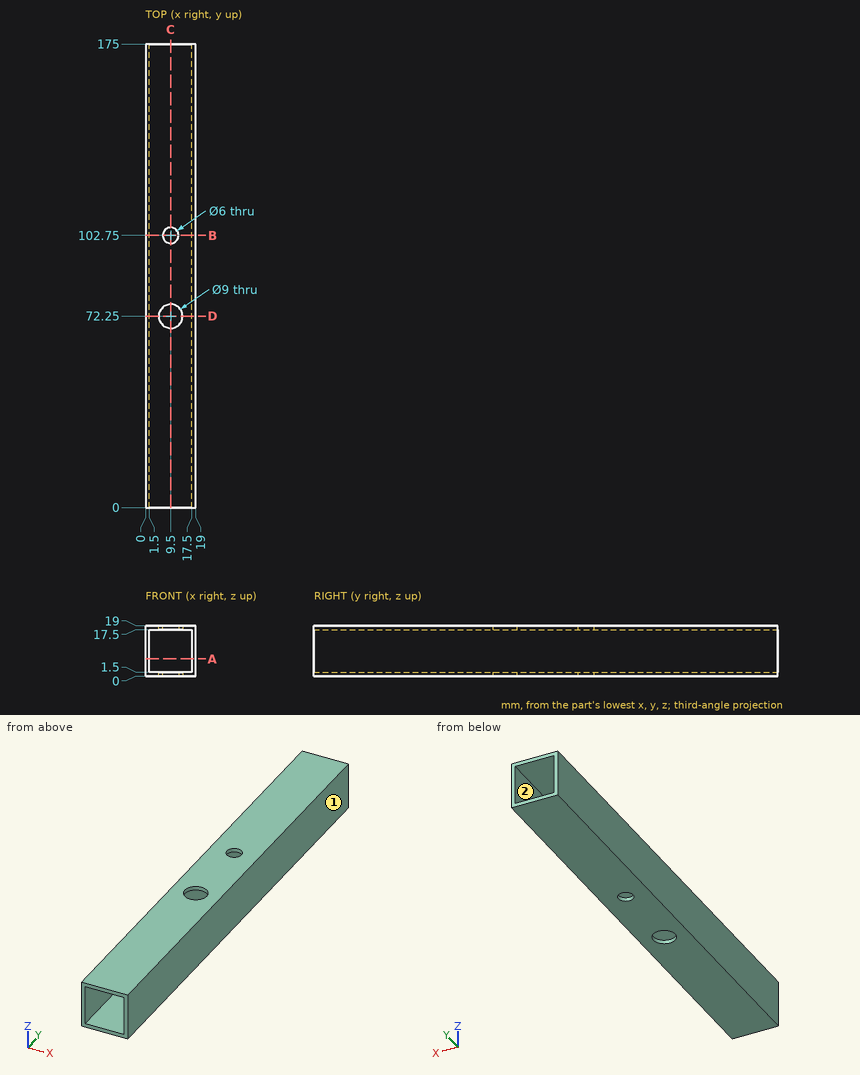
Source: three-view drawing plus pictorial views. Frame: mm from the lowest corner of the part. A direction names the side the tool comes from. Give positions to 0.01 mm unless a question says otherwise; leave off trailing zeros. Write each loop counter-clockwise with the first axis right and the second up, starting at its lowest first coordinate (ties: lowest second). Pieces come first, ordered by that corner, then holes. Notation, with made-up numbers: (-11.5, 82) - (-0.5, 82) arc R26 cw to (-0.5, 113) - close; hole circle Ø1 at (79, 30). An arc over 180 degrees is marked (long way). Write item = value, one per line. Start each with the question number.
Q1. Material intervals for probe 1 along Y at (x, z) = (9.5, 18.25); probe 2 along X at (y, z) = (59.5, 17.25), sorted ascending.
Q2. Cut plane C-C, the plane x = 9.5. Return loops of the section in (y, z).
Q3. Cut plane B-B, the plane y = 102.75. Return loops of the section in (x, z).
Q4. Pin query (flat end, axial travel): pin 1 Ø3.5 at (x, y) = (9.5, 102.75) entering from -Z. Return the tip coordinate at first contact, or that it passes through.
Q5. Reachability of the marked faces 1 and 2 from +Z, -Z, +X, -X, +Y, -Y: full face, straight path, thin tool, end or side. Return the list, or none.
Q6. Cut plane A-A, the plane z = 6.5. Return loops of the section in (x, y).
Q7. Cut plane D-D, the plane y = 72.25. Return loops of the section in (x, z).
Computed values:
q1.probe_1 = 0 to 67.75, 76.75 to 99.75, 105.75 to 175
q1.probe_2 = 0 to 1.5, 17.5 to 19
q2.outline = (0, 0) - (67.75, 0) - (67.75, 1.5) - (0, 1.5) - close; (0, 17.5) - (67.75, 17.5) - (67.75, 19) - (0, 19) - close; (76.75, 0) - (99.75, 0) - (99.75, 1.5) - (76.75, 1.5) - close; (76.75, 17.5) - (99.75, 17.5) - (99.75, 19) - (76.75, 19) - close; (105.75, 0) - (175, 0) - (175, 1.5) - (105.75, 1.5) - close; (105.75, 17.5) - (175, 17.5) - (175, 19) - (105.75, 19) - close
q3.outline = (0, 0) - (6.5, 0) - (6.5, 1.5) - (1.5, 1.5) - (1.5, 17.5) - (6.5, 17.5) - (6.5, 19) - (0, 19) - close; (12.5, 0) - (19, 0) - (19, 19) - (12.5, 19) - (12.5, 17.5) - (17.5, 17.5) - (17.5, 1.5) - (12.5, 1.5) - close
q4.pin_1 = through
q5.face_1 = +Z, -Z, +X, +Y, -Y
q5.face_2 = +Y, -Y
q6.outline = (0, 0) - (1.5, 0) - (1.5, 175) - (0, 175) - close; (17.5, 0) - (19, 0) - (19, 175) - (17.5, 175) - close
q7.outline = (0, 0) - (5, 0) - (5, 1.5) - (1.5, 1.5) - (1.5, 17.5) - (5, 17.5) - (5, 19) - (0, 19) - close; (14, 0) - (19, 0) - (19, 19) - (14, 19) - (14, 17.5) - (17.5, 17.5) - (17.5, 1.5) - (14, 1.5) - close
